For this review, take the finished solid that the model builds, in its own axes (mm). A direction names the side the tool comes from. Give positions to 0.01 mm unless a question says otherwise; leave off trailing zeros. Loops run counter-clockwise (first coordinate to the right, second up) from the corner with the lowest first, then second, coordinate; pieces in that order, holes last.
Autodesk Inventor part; units mm, degrees
ref_plane "YZ Plane" through (0, 0, 0) normal (1, 0, 0) x (0, 1, 0)
ref_plane "XZ Plane" through (0, 0, 0) normal (0, 1, 0) x (-1, 0, 0)
ref_plane "XY Plane" through (0, 0, 0) normal (0, 0, 1) x (1, 0, 0)
sketch "Sketch1" plane through (0, 0, 0) normal (0, 1, 0) x (-1, 0, 0)
  point P0 (0, 0)
sketch "Sketch2" plane through (0, 0, 0) normal (0, 1, 0) x (-1, 0, 0)
  line L0 (-4, 4) -> (4, 4)
  line L1 (4, 4) -> (4, -4)
  line L2 (4, -4) -> (-4, -4)
  line L3 (-4, -4) -> (-4, 4)
  line L4 (-4, 4) -> (4, -4) construction
  line L5 (4, 4) -> (-4, -4) construction
  point P0 (0, 0)
  dimension "d0" = 8
  dimension "d1" = 8
extrude "Extrusion1" add sketch "Sketch2" along normal blind 8
sketch "Sketch3" plane through (-4, 0, -4) normal (-1, 0, 0) x (0, 0, 1)
  line L0 (0, 1) -> (7, 1)
  line L1 (7, 1) -> (7, 7)
  line L2 (7, 7) -> (0, 7)
  line L3 (0, 7) -> (0, 1)
  line L4 (8, 0) -> (0, 0)
  line L5 (0, 0) -> (0, 8)
  point P0 (4, 0)
  dimension "d4" = 7
  dimension "d5" = 6
  dimension "d6" = 1
  dimension "d7" = 0
extrude "Extrusion2" cut sketch "Sketch3" against normal blind 7
sketch "Sketch4" plane through (-4, 0, 4) normal (0, 0, 1) x (1, 0, 0)
  circle A0 centre (2, 2) radius 1
  line L0 (8, 0) -> (0, 0)
  line L1 (8, 0) -> (8, 8)
  point P0 (4, 0)
  dimension "d10" = 2
  dimension "d11" = 2
  dimension "d12" = 6
sketch "Sketch5" plane through (4, 0, 4) normal (1, 0, 0) x (0, 0, -1)
  circle A0 centre (2, 6) radius 1
  line L0 (0, 0) -> (0, 8)
  line L1 (8, 0) -> (0, 0)
  point P0 (4, 0)
  dimension "d13" = 2
  dimension "d14" = 2
  dimension "d15" = 6
sketch "Sketch6" plane through (0, 0, 0) normal (0, -1, 0) x (1, 0, 0)
  circle A0 centre (2, -2) radius 1
  line L0 (4, 4) -> (-4, 4)
  line L1 (4, -4) -> (4, 4)
  point P0 (0, 0)
  dimension "d16" = 2
  dimension "d17" = 6
  dimension "d18" = 2
extrude "Extrusion3" cut sketch "Sketch6" against normal blind 1
extrude "Extrusion4" cut sketch "Sketch5" against normal blind 1
extrude "Extrusion5" cut sketch "Sketch4" against normal blind 1
sketch "Sketch7" plane through (0, 8, 0) normal (0, 1, 0) x (1, 0, 0)
  circle A0 centre (0, 0) radius 1
  line L0 (4, 4) -> (-4, 4)
  line L1 (-4, 4) -> (-4, -4)
  dimension "d25" = 2
  dimension "d26" = 4
  dimension "d27" = 4
extrude "Extrusion6" cut sketch "Sketch7" against normal blind 1
properties part number "Corner" material "Aluminum 6061"
Item 1: Clearance check with flat-ended pins moving along their axes: pin 1 Ø0.8 at (y, z) = (6.5, 2.5) entering from -X; pin 2 Ø1.6 at (x, y) = (-2, 2) entering from -Z. State where each tip first meets the part, or that it passes through.
Answer:
pin 1: stops at x = 3
pin 2: passes through
Item 2: Take a section at C-C on z = 0.5. Give the boundary of the cut face in (x, y), and give its area (3 significant figures).
Answer:
outline: (-4, 0) - (4, 0) - (4, 8) - (0.87, 8) - (0.87, 7) - (3, 7) - (3, 1) - (-4, 1) - close; (-4, 7) - (-0.87, 7) - (-0.87, 8) - (-4, 8) - close
area: 20.3 mm2
Item 3: The part is to be moulded in two halves that separate along Y. For faces 4 (the flat face through (1, 8, 1)), 5 (the flat face through (3.2, 4.3, -4)), 6 (the flat face through (3, 6.84, 2.79)), say which applies: released by +Y, released by -Y, zero draft, split by the parting line, or undercut.
Answer:
face 4: released by +Y
face 5: zero draft
face 6: undercut
Item 4: Take a section at B-B on y = 2.5. Give the boundary of the cut face in (x, z), and give its area (3 significant figures).
Answer:
outline: (-4, 3) - (-2.87, 3) - (-2.87, 4) - (-4, 4) - close; (-1.13, 3) - (3, 3) - (3, -4) - (4, -4) - (4, 4) - (-1.13, 4) - close
area: 13.3 mm2
Item 5: Take a section at A-A on x = 0. Give the boundary of the cut face in (y, z), and give its area (3 significant figures).
Answer:
outline: (0, -4) - (1, -4) - (1, 3) - (7, 3) - (7, 1) - (8, 1) - (8, 4) - (0, 4) - close; (7, -4) - (8, -4) - (8, -1) - (7, -1) - close
area: 20.0 mm2
Item 6: Take a section at D-D on z = 3.25. Give the boundary of the cut face in (x, y).
Answer:
outline: (-4, 0) - (4, 0) - (4, 8) - (-4, 8) - close; hole circle Ø2 at (-2, 2)
Item 7: For L1, parallel to Z at x = 3.5, y = 6; L2, parallel to Y at x = 3.4, z = 2; L3, parallel to Y at x = -1.25, z = -3, list the stretches that pass through material, from the lowest coordinate up.
Answer:
L1: z = -4 to 1, 3 to 4
L2: y = 0 to 5, 7 to 8
L3: y = 0 to 1, 7 to 8
Item 8: Tool access review of faces 1 (the cylindrical face through (1.2, 0.5, -2.6)), 2 (the flat face through (-1, 4, 3)), 3 (the cylindrical face through (-0.217, 7.507, 0.976)): name each direction out of +Z, -Z, +X, -X, +Y, -Y from which nothing blocks a thin tool from reaching the whole face with its end or side.
Answer:
face 1: -Y
face 2: -Z, -X
face 3: +Y
